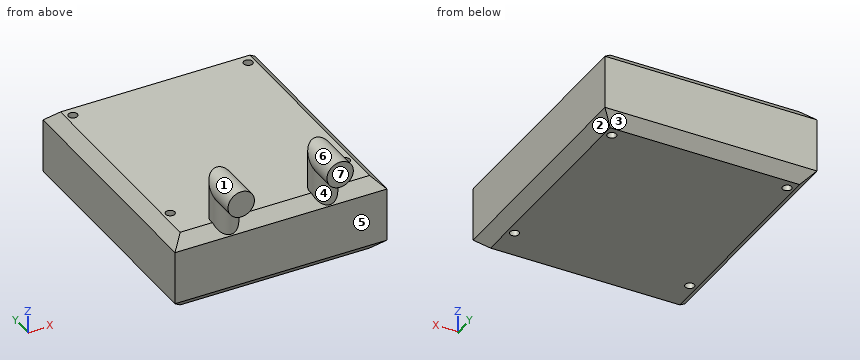
from build123d import *

# Parameters (mm, degrees)
SKETCH1_W           = 150
SKETCH1_H           = 171
BOSS_EXTRUDE1_DEPTH = 54
SKETCH2_R           = 3.175
CUT_EXTRUDE1_DEPTH  = 5.08
CHAMFER1_SIZE       = 8
SKETCH5_R           = 9.35


with BuildPart() as part:
    # Sketch1 → Boss-Extrude1 (new body)
    with BuildSketch(Plane.XY):
        Rectangle(SKETCH1_W, SKETCH1_H)
    extrude(amount=BOSS_EXTRUDE1_DEPTH)

    # Sketch2 → Cut-Extrude1 (cut)
    with BuildSketch(Plane.XY.offset(54)):
        with Locations((-62, 70.5)):
            Circle(SKETCH2_R)
        with Locations((62, 70.5)):
            Circle(SKETCH2_R)
        with Locations((62, -55.5)):
            Circle(SKETCH2_R)
        with Locations((-62, -55.5)):
            Circle(SKETCH2_R)
    cut_extrude1 = extrude(amount=-CUT_EXTRUDE1_DEPTH, mode=Mode.SUBTRACT)

    # Mirror1: Cut-Extrude1 across plane
    add(cut_extrude1.mirror(Plane.XY.offset(27)), mode=Mode.SUBTRACT)

    # Chamfer1
    chamfer1_edges = [part.edges().sort_by_distance(p)[0] for p in [
        (75, 0, 54),
        (0, -85.5, 54),
        (-75, 0, 54),
        (0, -85.5, 0),
        (75, 0, 0),
        (0, 85.5, 0),
        (-75, 0, 0),
        (0, 85.5, 54),
    ]]
    chamfer(chamfer1_edges, length=CHAMFER1_SIZE)

    # Sweep1: sweep along a path in Sketch6
    with BuildLine(Plane.ZY.offset(35)) as sweep1_path:
        Line((76.5, -98), (76.5, -75.5))
        Line((76.5, -75.5), (54, -75.5))
        Line((54, -75.5), (44, -75.5))
    # Sketch5 → Sweep1 (sweep)
    with BuildSketch(Plane.XY.offset(54)):
        with Locations((-35, -75.5)):
            Circle(SKETCH5_R)
    sweep1 = sweep(path=sweep1_path.line, transition=Transition.RIGHT)

    # Mirror2: Sweep1 across plane
    add(sweep1.mirror(Plane.ZY))


solid = part.part
The model under review builds one solid part; all positions refer to its coordinate system, in mm. Face numbers are marked on the shaded views. A direction names the side the tool comes from. Round coordinates to 2 decimals unless told otherwise and drop trailing zeros. Loops run counter-clockwise (first coordinate to the right, second up) from the corner with the lowest first, then second, coordinate; pieces in that order, holes last. Notation, with made-up numbers: M -15,13.5 L 34,13.5 A33 ccw 34,44.5 Z; hole C 42.5,-39.5 d10. An arc over 180 degrees is marked long. Answer as CSV lines item,"result". Start each with the question number.
Item 1: Wall thickness on line 1 (Z direction, x = -16, y = 45.5); line 2 (X direction, y = -55, z = 52); line 3 (Y direction, x = 15.5, z = 18.5): over which ranges is each line inside the solid? List them lowest first. Write a range as [from, to].
Item 2: For the marked faces 4, 5, 6 and 7, list the 3-axis set-ups (+Z, -Z, +X, -X, +Y, -Y) from which the entire face can be reached by the end or side of a thin tool; tool diameter is ignored.
Item 3: Consider section D-D (z = 26). Write out the cut boundary in (x, y), then the cut area to 4 significant figures.
Item 4: Mouldability with a two-part tool opening along X and no side actions: class the marked faces 1, 2 and 3 as released by +X, released by -X, zero draft, split by the parting line, or undercut.
Item 5: Consider section B-B (y = -34). Write out the cut boundary in (x, z), then the cut area to 3 significant figures.
Item 6: Consider section A-A (z = 80.5). Write out the cut boundary in (x, y), then the cut area to 3 significant figures.
Item 7: Consider section C-C (x = 35). Write out the cut boundary in (y, z).
Item 8: Insertion check: P1, Ø19, axis at x = -33.5, z = 17.5, coming from the -Y side; P2, Ø5.5, axis at x = -62, y = 70.5, coming from the -Z side; P3, Ø5, axis at x = -61, y = 70.5, coming from the +Z side. Each pin has a flat end and moves straight along its axis. Give the tip position at first contact, or say it passes through.
Answer:
1,line 1,"z = [0, 54]"
1,line 2,"x = [-69, -65.14], [-58.86, 58.86], [65.14, 69]"
1,line 3,"y = [-85.5, 85.5]"
2,face 4,"none"
2,face 5,"-Z, +X, -X, -Y"
2,face 6,"-Y"
2,face 7,"+Z, -Z, +X, -X, -Y"
3,outline,"M -75,-85.5 L 75,-85.5 L 75,85.5 L -75,85.5 Z"
3,area,"25,650 mm^2"
4,face 1,"undercut"
4,face 2,"released by +X"
4,face 3,"zero draft"
5,outline,"M -75,8 L -67,0 L 67,0 L 75,8 L 75,46 L 67,54 L -67,54 L -75,46 Z"
5,area,"7,970 mm^2"
6,outline,"M -43.45,-98 L -26.55,-98 L -26.55,-71.5 A9.35 ccw -43.45,-71.5 Z; M 26.55,-98 L 43.45,-98 L 43.45,-71.5 A9.35 ccw 26.55,-71.5 Z"
6,area,"1,030 mm^2"
7,outline,"M -98,67.15 L -84.85,67.15 L -84.85,46.65 L -85.5,46 L -85.5,8 L -77.5,0 L 77.5,0 L 85.5,8 L 85.5,46 L 77.5,54 L -66.15,54 L -66.15,85.85 L -98,85.85 Z"
8,P1,"stops at y = -85.5"
8,P2,"stops at z = 5.08"
8,P3,"stops at z = 54"
